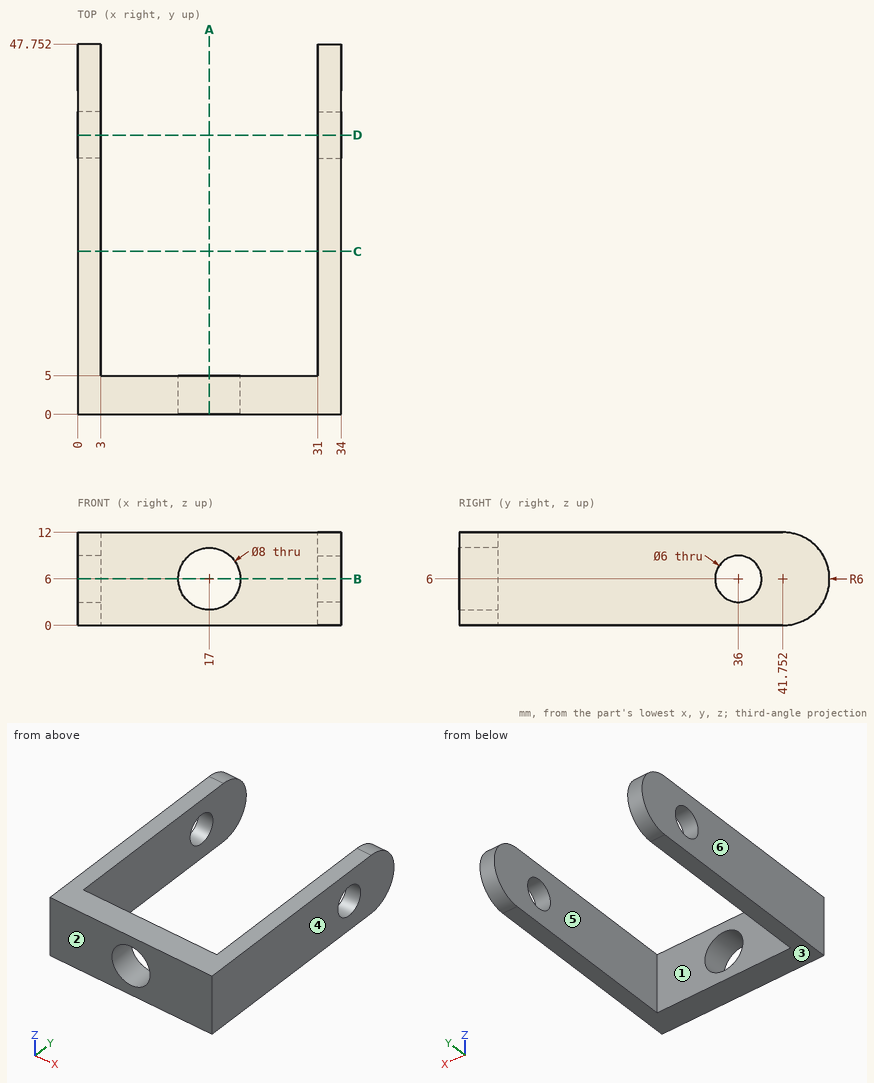
For this review, use the dimensioned drawing (mm, ordinates from the lowest corner) and the shaded views. A direction names the side the tool comes from. Coordinates: 2 decimals unless noted, no trailing zeros. Loops run counter-clockwise (first coordinate to the right, second up) from the corner with the lowest first, then second, coordinate; pieces in that order, holes last. Notation, with made-up numbers: (-1, 23) - (9, 23) arc R20 cw to (9, 43) - close; hole circle Ø5 at (82, 79). An arc over 180 degrees is marked (long way). Use CSV: the item, a comma, the result in double quotes. Start each with the question number.
1) Consider section D-D on y = 36. Write out the cut boundary in (x, z), then the cut area to 3 significant figures.
2) Consider section B-B on z = 6. Write out the cut boundary in (x, y).
3) Consider section C-C on y = 21. Write out the cut boundary in (x, z).
4) Consider section A-A on x = 17. Write out the cut boundary in (y, z).
5) For pin 1 Ø3 at (x, z) = (14, 9.5) entering from +Y; pin 2 Ø12 at (x, y) = (13.5, 34.5) entering from -Z, all flat-tipped, find the tip position at first contact; note any pin that passes through.
6) Wall thickness on L1, parallel to X at y = 1.1, z = 6; L2, parallel to X at y = 25.5, z = 1.5; L3, parallel to Y at x = 32.85, z = 6: over which ranges is each line inside the solid? List them lowest first. Write a range as from..to.
7) The part is to be moulded in two halves that separate along X. For the marked faces 3, 4, 5 and 6, say which applies: +X half, -X half, draft (parallel to the pull), parting line (faces both ways), or undercut.
8) Tool access review of the marked faces 1 and 2: name each direction out of +Z, -Z, +X, -X, +Y, -Y from which nothing blocks a thin tool from reaching the whole face with its end or side.
Geometry says:
1,outline,"(0, 0) - (3, 0) - (3, 3) - (0, 3) - close; (0, 9) - (3, 9) - (3, 12) - (0, 12) - close; (31, 0) - (34, 0) - (34, 3) - (31, 3) - close; (31, 9) - (34, 9) - (34, 12) - (31, 12) - close"
1,area,"36.0 mm^2"
2,outline,"(0, 0) - (13, 0) - (13, 5) - (3, 5) - (3, 33) - (0, 33) - close; (0, 39) - (3, 39) - (3, 47.75) - (0, 47.75) - close; (21, 0) - (34, 0) - (34, 33) - (31, 33) - (31, 5) - (21, 5) - close; (31, 39) - (34, 39) - (34, 47.75) - (31, 47.75) - close"
3,outline,"(0, 0) - (3, 0) - (3, 12) - (0, 12) - close; (31, 0) - (34, 0) - (34, 12) - (31, 12) - close"
4,outline,"(0, 0) - (5, 0) - (5, 2) - (0, 2) - close; (0, 10) - (5, 10) - (5, 12) - (0, 12) - close"
5,pin 1,"y = 5"
5,pin 2,"through"
6,L1,"0..13, 21..34"
6,L2,"0..3, 31..34"
6,L3,"0..33, 39..47.75"
7,face 3,"draft"
7,face 4,"+X half"
7,face 5,"undercut"
7,face 6,"-X half"
8,face 1,"+Z, -Z, +Y"
8,face 2,"+Z, -Z, +X, -X, -Y"
